Here's how the part is built. I have some questions about the finished solid (model axes, mm). A direction names the side the tool comes from. Round coordinates to 2 decimals unless told otherwise and drop trailing zeros. Loops run counter-clockwise (first coordinate to the right, second up) from the corner with the lowest first, then second, coordinate; pieces in that order, holes last. Notation, with made-up numbers: M 81,39.25 L 118,39.25 A20 cw 118,60.25 Z; hole C -33,42.25 d10. An arc over 180 degrees is marked long. Answer as a JSON object with one key per item and string values.
from build123d import *

# Parameters (mm, degrees)
SKETCH1_R           = 90
SKETCH1_R_2         = 9.7
SKETCH1_R_3         = 2
BOSS_EXTRUDE1_DEPTH = 3.5
CHAMFER1_SIZE       = 0.5


with BuildPart() as part:
    # Sketch1 → Boss-Extrude1 (new body)
    with BuildSketch(Plane(origin=(0, 0, 0), x_dir=(1, 0, 0), z_dir=(0, 1, 0))):
        Circle(SKETCH1_R)
        with Locations((-41.7, 41.7)):
            Circle(SKETCH1_R_2, mode=Mode.SUBTRACT)
        with Locations((41.7, 41.7)):
            Circle(SKETCH1_R_2, mode=Mode.SUBTRACT)
        with Locations((41.7, -41.7)):
            Circle(SKETCH1_R_2, mode=Mode.SUBTRACT)
        with Locations((-41.7, -41.7)):
            Circle(SKETCH1_R_2, mode=Mode.SUBTRACT)
        with Locations((-56.568542495, 56.568542495)):
            Circle(SKETCH1_R_3, mode=Mode.SUBTRACT)
        with Locations((-56.568542495, -56.568542495)):
            Circle(SKETCH1_R_3, mode=Mode.SUBTRACT)
        with Locations((56.568542495, 56.568542495)):
            Circle(SKETCH1_R_3, mode=Mode.SUBTRACT)
        with Locations((56.568542495, -56.568542495)):
            Circle(SKETCH1_R_3, mode=Mode.SUBTRACT)
        with Locations((-13.788582233, 20.859650045)):
            Circle(SKETCH1_R_3, mode=Mode.SUBTRACT)
        with Locations((20.859650045, -13.788582233)):
            Circle(SKETCH1_R_3, mode=Mode.SUBTRACT)
        with Locations((13.788582233, -20.859650045)):
            Circle(SKETCH1_R_3, mode=Mode.SUBTRACT)
        with Locations((-20.859650045, 13.788582233)):
            Circle(SKETCH1_R_3, mode=Mode.SUBTRACT)
        Polygon((7.14177849, -21.637467504), (-21.637467504, 7.14177849), (-7.14177849, 21.637467504), (21.637467504, -7.14177849), align=None, mode=Mode.SUBTRACT)
    extrude(amount=BOSS_EXTRUDE1_DEPTH)

    # Chamfer1
    chamfer1_edges = [part.edges().sort_by_distance(p)[0] for p in [
        (-90, 3.5, 0),
    ]]
    chamfer(chamfer1_edges, length=CHAMFER1_SIZE)


solid = part.part
Item 1: I want a section at B-B, the plane y = 2.1. State how many separate pieces and enclosed holes the cut face has, then the cut area to 3 significant figures.
Resolved:
{"separate pieces": "1", "enclosed holes": "13", "area": "23,300 mm²"}
Item 2: On a 3-axis mill with a long thin cutter (end or side, diameter ignored), from which of +Z, -Z, +X, -X, +Y, -Y can I reach the whole of each face in a straight line? I mean faces 1 (the face through (14.49, 1.73, 14.29)), 2 (the face through (-1, 0, 19)). Say none if no direction works.
Resolved:
{"face 1": "+Y, -Y", "face 2": "+Z, -Z, +X, -X, -Y"}
Item 3: If we mould it in two halves opening along X, with no side actions, what happens to faces 3 (the face through (19, 3.5, -1)), 4 (the face through (41.53, 1.479, 79.845)), 5 (the face through (46.176, 1.726, -33.094))? For each: pulls with the +X half, pulls with the -X half, needs draft (parallel to the pull), parting line crosses it, or undercut.
Resolved:
{"face 3": "needs draft", "face 4": "parting line crosses it", "face 5": "undercut"}
Item 4: I want a section at A-A, the plane x = 0. Please give me the cut outline in (y, z), then the cut area to 3 significant figures.
Resolved:
{"outline": "M 0,-90 L 3,-90 L 3.5,-89.5 L 3.5,-14.5 L 0,-14.5 Z; M 0,14.5 L 3.5,14.5 L 3.5,89.5 L 3,90 L 0,90 Z", "area": "528 mm²"}
Item 5: Please list where these lines run through material, in increasing order: probe 1 along X at (y, z) = (1.35, -40); probe 2 along X at (y, z) = (2.35, 57); probe 3 along Z at (x, y) = (46, 1.65). Write a range as from..to.
Resolved:
{"probe 1": "-80.62..-51.25, -32.15..32.15, 51.25..80.62", "probe 2": "-69.65..-58.52, -54.62..54.62, 58.52..69.65", "probe 3": "-77.36..-50.39, -33.01..33.01, 50.39..77.36"}
Item 6: I want a section at C-C, the plane z = 0. Please give me the cut outline in (x, y), then the cut area to 3 significant figures.
Resolved:
{"outline": "M -90,0 L -14.5,0 L -14.5,3.5 L -89.5,3.5 L -90,3 Z; M 14.5,0 L 90,0 L 90,3 L 89.5,3.5 L 14.5,3.5 Z", "area": "528 mm²"}
Item 7: I'm going to push a flat-ended pin straight in: pin 1 Ø25 at (x, z) = (-41.7, 41.7) entering from +Y. Where does the tip first touch, or does it pass through?
Resolved:
{"pin 1": "y = 3.5"}
